Autodesk Fusion 360 part; units mm, degrees
sketch "Sketch1" plane through (0, 0, 0) normal (0, 1, 0) x (1, 0, 0)
  line L0 (-8.9, 26.75) -> (8.9, 26.75)
  line L1 (8.9, 26.75) -> (8.9, -26.75)
  line L2 (8.9, -26.75) -> (-8.9, -26.75)
  line L3 (-8.9, -26.75) -> (-8.9, 26.75)
  line L4 (-8.9, 26.75) -> (8.9, -26.75) construction
  line L5 (8.9, 26.75) -> (-8.9, -26.75) construction
  dimension "d1" = 17.8
  dimension "d2" = 53.5
extrude "Extrude4" add sketch "Sketch1" along normal blind 1.6 makes body 1
extrude "Extrude1" add sketch "Sketch1" along normal blind 1.6 separate body makes body 2
sketch "Sketch2" plane through (0, 1.6, 0) normal (0, 1, 0) x (-1, 0, 0)
  line L0 (8.9, 26.75) -> (-8.9, 26.75)
  line L1 (-8.9, 26.75) -> (-8.9, -26.75)
  line L2 (-8.9, -26.75) -> (8.9, -26.75)
  line L3 (8.9, -26.75) -> (8.9, 26.75)
  line L4 (8.9, -26.75) -> (5.7, -26.75)
  line L5 (5.7, -26.75) -> (5.7, -23.55)
  line L6 (5.7, -23.55) -> (8.9, -23.55)
  line L7 (8.9, -23.55) -> (8.9, -26.75)
  line L8 (-5.65, -26.75) -> (-8.85, -26.75)
  line L9 (-8.85, -26.75) -> (-8.85, -23.55)
  line L10 (-8.85, -23.55) -> (-5.65, -23.55)
  line L11 (-5.65, -23.55) -> (-5.65, -26.75)
  line L12 (8.9, 24.05) -> (5.7, 24.05)
  line L13 (5.7, 24.05) -> (5.7, 27.25)
  line L14 (5.7, 27.25) -> (8.9, 27.25)
  line L15 (8.9, 27.25) -> (8.9, 24.05)
  line L16 (-5.65, 24.05) -> (-8.85, 24.05)
  line L17 (-8.85, 24.05) -> (-8.85, 27.25)
  line L18 (-8.85, 27.25) -> (-5.65, 27.25)
  line L19 (-5.65, 27.25) -> (-5.65, 24.05)
  point P0 (-5.65, -26.75)
  point P1 (8.9, 24.05)
  point P2 (-5.65, 24.05)
  dimension "d7" = 3.2
  dimension "d8" = 3.2
  dimension "d11" = -14.55
  dimension "d12" = 50.8
  dimension "d13" = 38.8
sketch "Sketch4" plane through (0, 1.6, 0) normal (0, 1, 0) x (-1, 0, 0)
  line L0 (8.9, 26.75) -> (-8.9, 26.75)
  line L1 (-8.9, 26.75) -> (-8.9, -26.75)
  line L2 (-8.9, -26.75) -> (8.9, -26.75)
  line L3 (8.9, -26.75) -> (8.9, 26.75)
  line L4 (8.9, -26.75) -> (5.7, -26.75)
  line L5 (5.7, -26.75) -> (5.7, -23.55)
  line L6 (5.7, -23.55) -> (8.9, -23.55)
  line L7 (8.9, -23.55) -> (8.9, -26.75)
  line L8 (-8.9, -26.75) -> (-8.9, -23.55)
  line L9 (-8.9, -23.55) -> (-5.7, -23.55)
  line L10 (-5.7, -26.75) -> (-8.9, -26.75)
  line L11 (-5.7, -23.55) -> (-5.7, -26.75)
  line L12 (5.7, 23.55) -> (5.7, 26.75)
  line L13 (5.7, 26.75) -> (8.9, 26.75)
  line L14 (8.9, 23.55) -> (5.7, 23.55)
  line L15 (8.9, 26.75) -> (8.9, 23.55)
  line L16 (-8.9, 23.55) -> (-8.9, 26.75)
  line L17 (-8.9, 26.75) -> (-5.7, 26.75)
  line L18 (-5.7, 23.55) -> (-8.9, 23.55)
  line L19 (-5.7, 26.75) -> (-5.7, 23.55)
  point P0 (8.9, -26.75)
  point P1 (-5.7, -26.75)
  point P2 (-5.7, -26.75)
  point P3 (8.9, 23.55)
  point P4 (8.9, 23.55)
  point P5 (-5.7, 23.55)
  point P6 (-5.7, 23.55)
  dimension "d24" = 3.2
  dimension "d25" = 3.2
  dimension "d28" = -14.6
  dimension "d29" = 50.3
extrude "Extrude5" add sketch "Sketch4" along normal blind 11.575 contours L0 L3 L12 L13 L14 L15 | L0 L1 L16 L17 L18 L19 | L2 L3 L4 L5 L6 L7 | L1 L2 L8 L9 L10 L11 bodies 1 2
sketch "Sketch5" plane through (0, 13.175, 0) normal (0, 1, 0) x (-1, 0, 0)
  line L0 (8.9, -23.55) -> (5.7, -23.55)
  line L1 (5.7, -23.55) -> (5.7, -26.75)
  line L2 (5.7, -26.75) -> (8.9, -26.75)
  line L3 (8.9, -26.75) -> (8.9, -23.55)
  line L4 (8.9, -26.75) -> (-8.9, -26.75)
  line L5 (-8.9, -26.75) -> (-8.9, 26.75)
  line L6 (-8.9, 26.75) -> (8.9, 26.75)
  line L7 (8.9, 26.75) -> (8.9, -26.75)
  point P0 (-8.9, 26.75)
extrude "Extrude6" add sketch "Sketch5" along normal blind 1.6 bodies 1
sketch "Sketch6" plane through (0, 14.775, 0) normal (0, 1, 0) x (-1, 0, 0)
  line L0 (8.9, 26.75) -> (-8.9, 26.75)
  line L1 (-8.9, 26.75) -> (-8.9, -26.75)
  line L2 (-8.9, -26.75) -> (8.9, -26.75)
  line L3 (8.9, -26.75) -> (8.9, 26.75)
  line L4 (8.9, 7.5) -> (-8.9, 7.5)
  line L5 (-8.9, 7.5) -> (-8.9, 9.1)
  line L6 (-8.9, 9.1) -> (8.9, 9.1)
  line L7 (8.9, 9.1) -> (8.9, 7.5)
  line L8 (8.9, -26.75) -> (-8.9, -26.75)
  dimension "d34" = 1.6
  dimension "d35" = 34.25
extrude "Extrude7" add sketch "Sketch6" along normal blind 3.3 contours L1 L3 L4 L5 L6 L7 bodies 1
sketch "Sketch7" plane through (0, 0, 7.5) normal (0, 0, -1) x (-1, 0, 0)
  line L0 (-8.9, 14.775) -> (8.9, 14.775)
  line L1 (8.9, 14.775) -> (8.9, 18.075)
  line L2 (8.9, 18.075) -> (-8.9, 18.075)
  line L3 (-8.9, 18.075) -> (-8.9, 14.775)
  line L4 (-8.9, 18.075) -> (8.9, 18.075)
  line L5 (8.9, 18.075) -> (8.9, 16.775)
  line L6 (8.9, 16.775) -> (-8.9, 16.775)
  line L7 (-8.9, 16.775) -> (-8.9, 18.075)
  dimension "d38" = 1.3
extrude "Extrude8" add sketch "Sketch7" along normal blind 2 contours L1 L2 L3 L4 L5 L6 L7 bodies 1
equation "d1 = boxWidth"
equation "d11 = -17.75 mm + 3.2 mm"
equation "d12 = 54 mm - 3.2 mm"
equation "BoxLength = 53.5 mm"
equation "boxWidth = 17.8 mm"
equation "d28 = -17.8 mm + 3.2 mm"
equation "d29 = 53.5 mm - 3.2 mm"
equation "d30 = 14.075 mm - 2.5 mm"
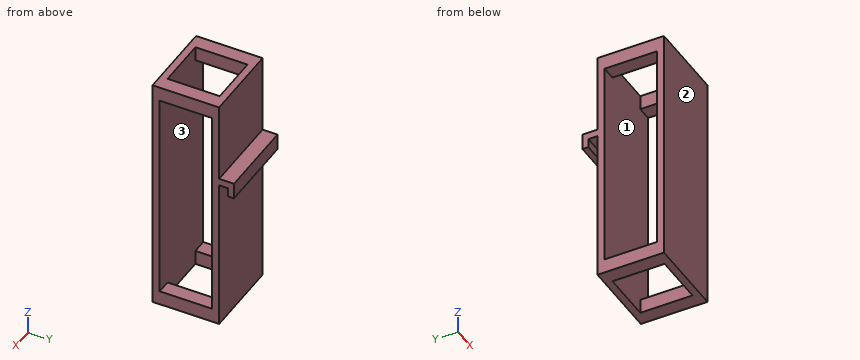
The listing builds one solid part. Answer for the finished solid, in the listing's coordinates (mm). Face numbers are marked on the shaded views. Coordinates: 2 decimals unless noted, no trailing zeros. Order: outer loops, then holes, each group sorted by start corner. A loop starts at its lowest first (then second) coordinate and runs counter-clockwise, first axis right, second up. Notation, with made-up numbers: (-36.5, 18) -> (-11.5, 18) arc R34 ccw to (-11.5, 48) -> close; hole circle Ø5 at (46, -38.5). An arc over 180 degrees is marked (long way). Answer in a Markdown table with one row per item. Add a question column.
Item 1: Find section D-D (x = -7). Write down the section's boundary in (y, z) (3 decimals).
Item 2: Find the intervals of material crossed by L1, parallel to Z at x = -8, y = 11.5; L2, parallel to Y at x = -7, z = -7.5 (3 decimals); L3, parallel to Y at x = 5.5, z = 9 (3 decimals), in increasing order. Write a range as from..to.
Item 3: Determine the mould class of the marked faces 1, 2 and 3 for opening direction Z: +Z half, -Z half, draft (parallel to the pull), parting line (faces both ways), or undercut.
Item 4: Find section B-B (z = -8.5). Write down the section's boundary in (x, y) (3 decimals), then the cut area to 3 significant figures.
Item 5: Find section C-C (x = 4.25). Write down the section's boundary in (y, z) (3 decimals).
Item 6: Each of these flat-tipped pins is pushed along its axis until it touches: P1, Ø0.6, axis at x = -4.5, y = 16, coming from the -Z side; P2, Ø5.5, axis at x = -3, z = -7, coming from the +Y side (3 decimals); P3, Ø0.7, axis at x = -3, y = 17.5, coming from the -Z side. Where does it stop, or does it pass through?
Item 7: Find section A-A (y = 2.25). Write down the section's boundary in (x, z), then the cut area to 3 significant figures.
Result set:
| question | item | result |
|---|---|---|
| 1 | outline | (0, -26.75) -> (14.775, -26.75) -> (14.775, 7.5) -> (16.775, 7.5) -> (16.775, 5.5) -> (18.075, 5.5) -> (18.075, 9.1) -> (14.775, 9.1) -> (14.775, 26.75) -> (0, 26.75) -> close; hole (1.6, -23.55) -> (13.175, -23.55) -> (13.175, 23.55) -> (1.6, 23.55) -> close |
| 2 | L1 | z = -26.75..-23.55, 23.55..26.75 |
| 2 | L2 | y = 0..1.6, 13.175..14.775 |
| 2 | L3 | y = 0..1.6, 13.175..18.075 |
| 3 | face 1 | undercut |
| 3 | face 2 | draft |
| 3 | face 3 | undercut |
| 4 | outline | (-8.9, 0) -> (8.9, 0) -> (8.9, 1.6) -> (-8.9, 1.6) -> close; (-8.9, 13.175) -> (8.9, 13.175) -> (8.9, 14.775) -> (-8.9, 14.775) -> close |
| 4 | area | 57.0 mm² |
| 5 | outline | (0, -26.75) -> (1.6, -26.75) -> (1.6, 26.75) -> (0, 26.75) -> close; (13.175, -26.75) -> (14.775, -26.75) -> (14.775, 7.5) -> (16.775, 7.5) -> (16.775, 5.5) -> (18.075, 5.5) -> (18.075, 9.1) -> (14.775, 9.1) -> (14.775, 26.75) -> (13.175, 26.75) -> close |
| 6 | P1 | stops at z = 7.5 |
| 6 | P2 | stops at y = 14.775 |
| 6 | P3 | stops at z = 5.5 |
| 7 | outline | (-8.9, -26.75) -> (-5.7, -26.75) -> (-5.7, -23.55) -> (-8.9, -23.55) -> close; (-8.9, 23.55) -> (-5.7, 23.55) -> (-5.7, 26.75) -> (-8.9, 26.75) -> close; (5.7, -26.75) -> (8.9, -26.75) -> (8.9, -23.55) -> (5.7, -23.55) -> close; (5.7, 23.55) -> (8.9, 23.55) -> (8.9, 26.75) -> (5.7, 26.75) -> close |
| 7 | area | 41.0 mm² |
